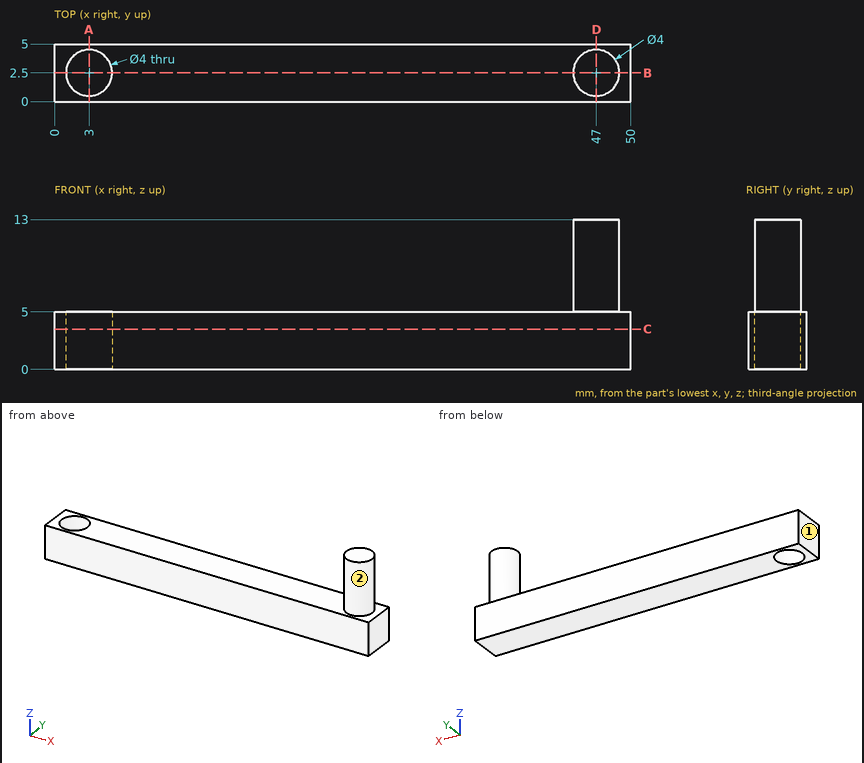
The drawing under review shows one solid part. Ordinate dimensions are in mm from its lowest x, y, z. A direction names the side the tool comes from. Coordinates: 2 decimals unless noted, no trailing zeros. Order: outer loops, then holes, each group sorted by start corner. A loop starts at its lowest first (then second) coordinate and runs counter-clockwise, first axis right, second up. Notation, with made-up numbers: (78, 41) -> (126, 41) arc R29 ccw to (126, 73) -> close; hole circle Ø4 at (55, 71.5). An arc over 180 degrees is marked (long way). Answer in a Markdown table with one row per item.
(1) Consider section C-C (z = 3.5). Write out the cut boundary in (x, y).
Answers:
| item | result |
|---|---|
| outline | (0, 0) -> (50, 0) -> (50, 5) -> (0, 5) -> close; hole circle Ø4 at (3, 2.5) |
(2) Consider section A-A (x = 3). Write out the cut boundary in (y, z), plus the area to 3 significant figures.
Answers:
| item | result |
|---|---|
| outline | (0, 0) -> (0.5, 0) -> (0.5, 5) -> (0, 5) -> close; (4.5, 0) -> (5, 0) -> (5, 5) -> (4.5, 5) -> close |
| area | 5.00 mm² |
(3) Consider section B-B (y = 2.5). Write out the cut boundary in (x, z), plus the area to 3 significant figures.
Answers:
| item | result |
|---|---|
| outline | (0, 0) -> (1, 0) -> (1, 5) -> (0, 5) -> close; (5, 0) -> (50, 0) -> (50, 5) -> (49, 5) -> (49, 13) -> (45, 13) -> (45, 5) -> (5, 5) -> close |
| area | 262 mm² |
(4) Machinability: for the marked faces 1 and 2, which of the approach directions +Z, -Z, +X, -X, +Y, -Y give a long, thin tool a straight path to every point of the face, cutting with its end or side? Answer none if there is none.
Answers:
| item | result |
|---|---|
| face 1 | +Z, -Z, -X, +Y, -Y |
| face 2 | +Z |
(5) Wall thickness on line 1 along Y through (x, z) = (3, 2.75); line 2 along Z through (x, y) = (6.5, 0.9); line 3 along X through (y, z) = (3.9, 12): over which ranges is each line inside the solid? List them lowest first.
Answers:
| item | result |
|---|---|
| line 1 | 0 to 0.5, 4.5 to 5 |
| line 2 | 0 to 5 |
| line 3 | 45.57 to 48.43 |
(6) Insertion check: pin 1 (1 mm diameter, centred on x = 34, y = 0.5, fed in from +Z); pin 2 (3 mm diameter, centred on x = 30.5, y = 1, fed in from -Z). Each pin has a flat end and moves straight along its axis. Give the tip position at first contact, or say it passes through.
Answers:
| item | result |
|---|---|
| pin 1 | z = 5 |
| pin 2 | z = 0 |
(7) Consider section D-D (x = 47). Write out the cut boundary in (y, z), plus the area to 3 significant figures.
Answers:
| item | result |
|---|---|
| outline | (0, 0) -> (5, 0) -> (5, 5) -> (4.5, 5) -> (4.5, 13) -> (0.5, 13) -> (0.5, 5) -> (0, 5) -> close |
| area | 57.0 mm² |
